from build123d import *

# Parameters (mm, degrees)
SKETCH_2_W      = 1040
SKETCH_2_H      = 530
EXTRUDE_1_DEPTH = 170
SKETCH_3_W      = 800
SKETCH_3_H      = 60
SKETCH_3_W_2    = 60
SKETCH_3_H_2    = 410
EXTRUDE_2_DEPTH = 60
SKETCH_4_W      = 60
SKETCH_4_H      = 60
EXTRUDE_3_DEPTH = 560
EXTRUDE_4_REACH = 1274.046
SKETCH_5_W      = 60
SKETCH_5_H      = 60
SKETCH_5_H_2    = 40
EXTRUDE_5_REACH = 1231.512
SKETCH_6_W      = 60
SKETCH_6_H      = 60
EXTRUDE_6_REACH = 1231.512
SKETCH_7_W      = 370
SKETCH_7_H      = 40


with BuildPart() as part:
    # ｽｹｯﾁ2 → ﾎﾞｽ - 押し出し1 (new body)
    with BuildSketch(Plane(origin=(0, 0, 0), x_dir=(1, 0, 0), z_dir=(0, 1, 0))):
        with Locations((520, 265)):
            Rectangle(SKETCH_2_W, SKETCH_2_H)
    extrude(amount=EXTRUDE_1_DEPTH)

    # ｽｹｯﾁ3 → ﾎﾞｽ - 押し出し2 (add)
    with BuildSketch(Plane(origin=(0, 0, 0), x_dir=(-1, 0, 0), z_dir=(0, -1, 0))):
        with Locations((-520, 420)):
            Rectangle(SKETCH_3_W, SKETCH_3_H)
        with Locations((-950, 265)):
            Rectangle(SKETCH_3_W_2, SKETCH_3_H_2)
        with Locations((-520, 110)):
            Rectangle(SKETCH_3_W, SKETCH_3_H)
        with Locations((-90, 265)):
            Rectangle(SKETCH_3_W_2, SKETCH_3_H_2)
    extrude(amount=EXTRUDE_2_DEPTH)

    # ｽｹｯﾁ4 → ﾎﾞｽ - 押し出し3 (add)
    with BuildSketch(Plane(origin=(0, -60, 0), x_dir=(-1, 0, 0), z_dir=(0, -1, 0))):
        with Locations((-950, 420)):
            Rectangle(SKETCH_4_W, SKETCH_4_H)
        with Locations((-950, 110)):
            Rectangle(SKETCH_4_W, SKETCH_4_H)
        with Locations((-90, 420)):
            Rectangle(SKETCH_4_W, SKETCH_4_H)
        with Locations((-90, 110)):
            Rectangle(SKETCH_4_W, SKETCH_4_H)
    extrude(amount=EXTRUDE_3_DEPTH)

    # ｽｹｯﾁ5 → ﾎﾞｽ - 押し出し4 (add, up to next)
    with BuildSketch(Plane(origin=(0, 0, -140), x_dir=(-1, 0, 0), z_dir=(0, 0, -1)), mode=Mode.PRIVATE) as extrude_4_sk1:
        with Locations((-90, -510)):
            Rectangle(SKETCH_5_W, SKETCH_5_H)
    extrude_4_tool1 = extrude(extrude_4_sk1.sketch, amount=EXTRUDE_4_REACH, mode=Mode.PRIVATE) - part.part
    # ｽｹｯﾁ5 → ﾎﾞｽ - 押し出し4 (add, up to next)
    with BuildSketch(Plane(origin=(0, 0, -140), x_dir=(-1, 0, 0), z_dir=(0, 0, -1)), mode=Mode.PRIVATE) as extrude_4_sk2:
        with Locations((-950, -510)):
            Rectangle(SKETCH_5_W, SKETCH_5_H)
    extrude_4_tool2 = extrude(extrude_4_sk2.sketch, amount=EXTRUDE_4_REACH, mode=Mode.PRIVATE) - part.part
    # ｽｹｯﾁ5 → ﾎﾞｽ - 押し出し4 (add, up to next)
    with BuildSketch(Plane(origin=(0, 0, -140), x_dir=(-1, 0, 0), z_dir=(0, 0, -1)), mode=Mode.PRIVATE) as extrude_4_sk3:
        with Locations((-950, -190)):
            Rectangle(SKETCH_5_W, SKETCH_5_H_2)
    extrude_4_tool3 = extrude(extrude_4_sk3.sketch, amount=EXTRUDE_4_REACH, mode=Mode.PRIVATE) - part.part
    # ｽｹｯﾁ5 → ﾎﾞｽ - 押し出し4 (add, up to next)
    with BuildSketch(Plane(origin=(0, 0, -140), x_dir=(-1, 0, 0), z_dir=(0, 0, -1)), mode=Mode.PRIVATE) as extrude_4_sk4:
        with Locations((-90, -190)):
            Rectangle(SKETCH_5_W, SKETCH_5_H_2)
    extrude_4_tool4 = extrude(extrude_4_sk4.sketch, amount=EXTRUDE_4_REACH, mode=Mode.PRIVATE) - part.part
    add(extrude_4_tool1.solids().sort_by_distance((90, -510, -140))[0])
    add(extrude_4_tool2.solids().sort_by_distance((950, -510, -140))[0])
    add(extrude_4_tool3.solids().sort_by_distance((950, -190, -140))[0])
    add(extrude_4_tool4.solids().sort_by_distance((90, -190, -140))[0])

    # ｽｹｯﾁ6 → ﾎﾞｽ - 押し出し5 (add, up to next)
    with BuildSketch(Plane(origin=(120, 0, 0), x_dir=(0, 0, -1), z_dir=(1, 0, 0)), mode=Mode.PRIVATE) as extrude_5_sk1:
        with Locations((420, -510)):
            Rectangle(SKETCH_6_W, SKETCH_6_H)
    extrude_5_tool1 = extrude(extrude_5_sk1.sketch, amount=EXTRUDE_5_REACH, mode=Mode.PRIVATE) - part.part
    # ｽｹｯﾁ6 → ﾎﾞｽ - 押し出し5 (add, up to next)
    with BuildSketch(Plane(origin=(120, 0, 0), x_dir=(0, 0, -1), z_dir=(1, 0, 0)), mode=Mode.PRIVATE) as extrude_5_sk2:
        with Locations((110, -510)):
            Rectangle(SKETCH_6_W, SKETCH_6_H)
    extrude_5_tool2 = extrude(extrude_5_sk2.sketch, amount=EXTRUDE_5_REACH, mode=Mode.PRIVATE) - part.part
    add(extrude_5_tool1.solids().sort_by_distance((120, -510, -420))[0])
    add(extrude_5_tool2.solids().sort_by_distance((120, -510, -110))[0])

    # ｽｹｯﾁ7 → ﾎﾞｽ - 押し出し6 (add, up to next)
    with BuildSketch(Plane(origin=(120, 0, 0), x_dir=(0, 0, -1), z_dir=(1, 0, 0)), mode=Mode.PRIVATE) as extrude_6_sk1:
        with Locations((265, -190)):
            Rectangle(SKETCH_7_W, SKETCH_7_H)
    extrude_6_tool1 = extrude(extrude_6_sk1.sketch, amount=EXTRUDE_6_REACH, mode=Mode.PRIVATE) - part.part
    add(extrude_6_tool1.solids().sort_by_distance((120, -190, -265))[0])


solid = part.part
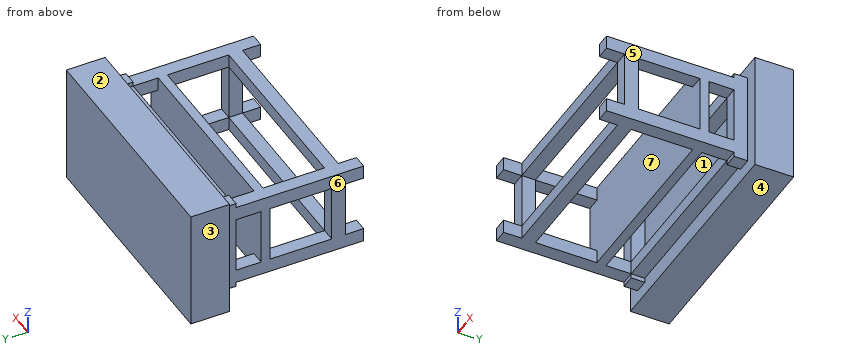
For this review, take the finished solid that the model builds, in its own axes (mm). Face numbers are marked on the shaded views. A direction names the side the tool comes from. Give positions to 0.01 mm unless a question says otherwise; leave off trailing zeros. Order: outer loops, then holes, each group sorted by start corner. A loop starts at its lowest first (then second) coordinate and runs counter-clockwise, first axis right, second up. Notation, with made-up numbers: (40.5, 37.25) - (74.5, 37.25) arc R29 ccw to (74.5, 72.25) - close; hole circle Ø5 at (48.25, 83.5). An arc over 180 degrees is marked (long way). Answer as a JSON object with one key per item and string values. Group by question number.
Item 1: Machinability: for the marked faces 4, 5, 6 and 7, which of the approach directions +Z, -Z, +X, -X, +Y, -Y give a long, thin tool a straight path to every point of the face, cutting with its end or side? Answer none if there is none.
Item 2: Take a section at D-D on y = -14. Give the boundary of the cut face in (x, z).
Item 3: Take a section at B-B on x = 146. Give the boundary of the cut face in (y, z), and give its area (3 significant figures).
Item 4: Clearance check with flat-ended pins moving along their axes: pin 1 Ø18 at (y, z) = (-367, -430) entering from +X; pin 2 Ø10 at (x, y) = (130.5, -206.5) entering from +Z; pin 3 Ø18 at (y, z) = (-95, -418.5) entering from -X. State where each tip first meets the part, or that it passes through.
Item 5: Wall thickness on line 1 along Y through (x, z) = (316, -89); line 2 along Y through (x, z) = (246.5, -184.5); line 3 along X through (y, z) = (-488, -227): over which ranges is each line inside the solid? List them lowest first.
Item 6: Take a section at A-A on y = -134. Give the boundary of the cut face in (x, z), and give its area (3 significant figures).
Item 7: Take a section at C-C on z = -99. Give the boundary of the cut face in (x, y), and give its area (3 significant figures).
Item 8: Draft analysis for pull direction Z (two halves, no side actions). For the marked faces 1, 2 and 3, state which applies: pulls with the +Z half, pulls with the -Z half, needs draft (parallel to the pull), parting line crosses it, or undercut.
Reported:
{
 "1": {"face 4": "-Z, +X, -X, +Y, -Y", "face 5": "+Z, -Z, +X, -Y", "face 6": "+Z, -Z, -X, -Y", "face 7": "none"},
 "2": {"outline": "(60, -470) - (120, -470) - (120, -450) - (920, -450) - (920, -470) - (980, -470) - (980, -60) - (920, -60) - (920, -80) - (120, -80) - (120, -60) - (60, -60) - close; hole (120, -390) - (920, -390) - (920, -140) - (120, -140) - close"},
 "3": {"outline": "(-540, -450) - (-480, -450) - (-480, -390) - (-540, -390) - close; (-540, -140) - (-480, -140) - (-480, -80) - (-540, -80) - close; (-210, -450) - (-170, -450) - (-170, -80) - (-210, -80) - close; (-60, -450) - (0, -450) - (0, -530) - (170, -530) - (170, 0) - (0, 0) - (0, -80) - (-60, -80) - (-60, -140) - (0, -140) - (0, -390) - (-60, -390) - close", "area": "119,000 mm^2"},
 "4": {"pin 1": "x = 980", "pin 2": "z = -80", "pin 3": "x = 60"},
 "5": {"line 1": "-540 to -480, -210 to -170, -60 to 170", "line 2": "-210 to -170, 0 to 170", "line 3": "60 to 120, 920 to 980"},
 "6": {"outline": "(60, -450) - (120, -450) - (120, -390) - (60, -390) - close; (60, -140) - (120, -140) - (120, -80) - (60, -80) - close; (920, -450) - (980, -450) - (980, -390) - (920, -390) - close; (920, -140) - (980, -140) - (980, -80) - (920, -80) - close", "area": "14,400 mm^2"},
 "7": {"outline": "(0, 0) - (60, 0) - (60, -620) - (120, -620) - (120, -540) - (920, -540) - (920, -620) - (980, -620) - (980, 0) - (1040, 0) - (1040, 170) - (0, 170) - close; hole (120, -480) - (920, -480) - (920, -210) - (120, -210) - close; hole (120, -170) - (920, -170) - (920, -60) - (120, -60) - close", "area": "379,000 mm^2"},
 "8": {"face 1": "undercut", "face 2": "pulls with the +Z half", "face 3": "needs draft"}
}
